Study the drawing (mm; zero at the part's minimum x, y, z) and answer. A direction names the side the tool comes from. Coordinates: 2 decimals unless noted, no trailing zeros. Order: outer loops, then holes, each group sorted by start corner. A loop starts at its lowest first (then second) coordinate and runs counter-clockwise, first axis right, second up.
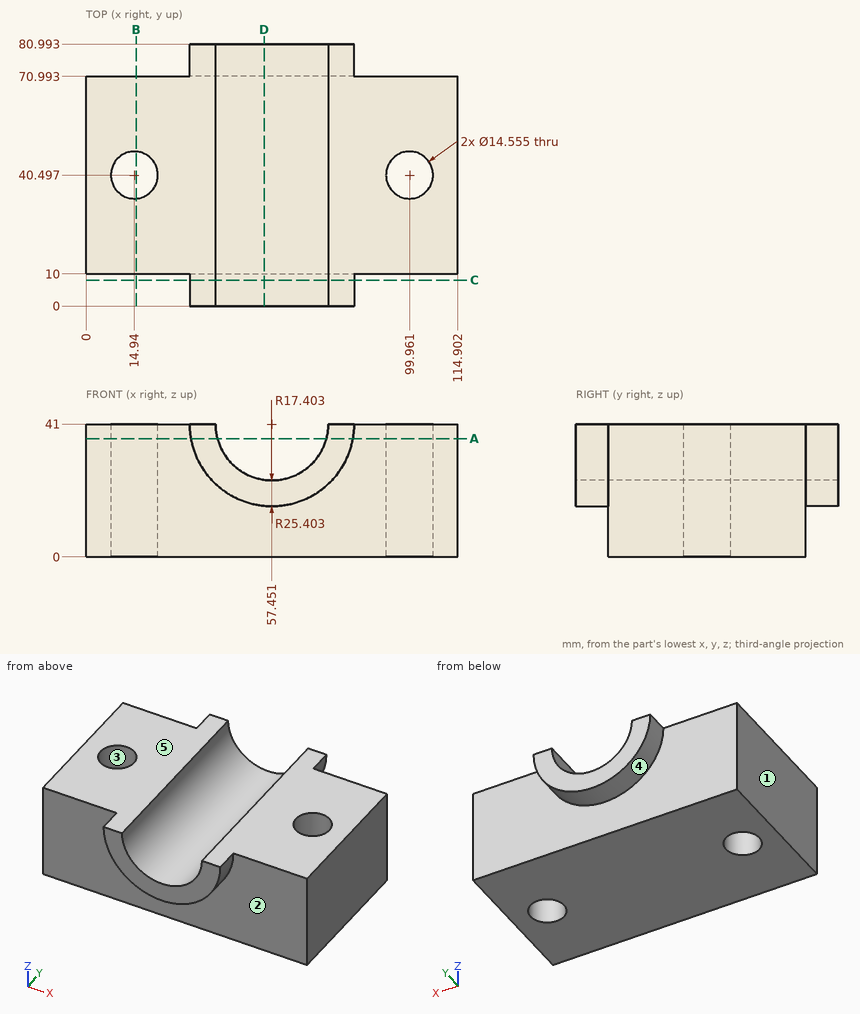
1) A cutting plane is placed at A-A, the plane z = 36.5. State how many separate pieces and enclosed holes the cut face has, and give its area (3 significant figures).
A:
separate pieces: 2
enclosed holes: 2
area: 4,950 mm2
2) Flat-ended cylindrical pins translate along their axes: pin 1 Ø1 at (x, y) = (67.5, 13.5) entering from -Z; pin 2 Ø10 at (x, z) = (91, 29) entering from +Y. Find the tip coordinate at first contact, or state that the pin passes through.
A:
pin 1: stops at z = 0
pin 2: stops at y = 70.99
3) A cutting plane is placed at C-C, the plane y = 8. Determine the outline of the cut face in (x, z).
A:
outline: (32.05, 41) arc R25.4 ccw to (82.85, 41) - (74.85, 41) arc R17.4 cw to (40.05, 41) - close
4) A cutting plane is placed at D-D, the plane x = 55. Determine the outline of the cut face in (y, z) (1 decimal), and give its area (3 significant figures).
A:
outline: (0, 15.7) - (10, 15.7) - (10, 0) - (71, 0) - (71, 15.7) - (81, 15.7) - (81, 23.8) - (0, 23.8) - close
area: 1,610 mm2
5) Which of the six approach directions +Z, -Z, +X, -X, +Y, -Y give full straight-line access (tool end or side, diameter ignored) to the marked faces 4 and 5?
A:
face 4: -Z, +Y
face 5: +Z, +X, -X, +Y, -Y
6) Determine the mould class of the marked faces 1, 2 and 3 for opening direction X: pulls with the +X half, pulls with the -X half, needs draft (parallel to the pull), parting line crosses it, or undercut.
A:
face 1: pulls with the -X half
face 2: needs draft
face 3: undercut
7) A cutting plane is placed at B-B, the plane x = 15.5. Determine the outline of the cut face in (y, z).
A:
outline: (10, 0) - (33.24, 0) - (33.24, 41) - (10, 41) - close; (47.75, 0) - (70.99, 0) - (70.99, 41) - (47.75, 41) - close
8) Straight lines are drawn through the part: line 1 (X direction, y = 40, z = 11); line 2 (Y direction, x = 7, z = 23.5); line 3 (X direction, y = 38.5, z = 9.5). For each, find the intervals that lie inside material, in ascending order.
A:
line 1: x = 0 to 7.68, 22.2 to 92.7, 107.22 to 114.9
line 2: y = 10 to 70.99
line 3: x = 0 to 7.94, 21.94 to 92.96, 106.96 to 114.9
